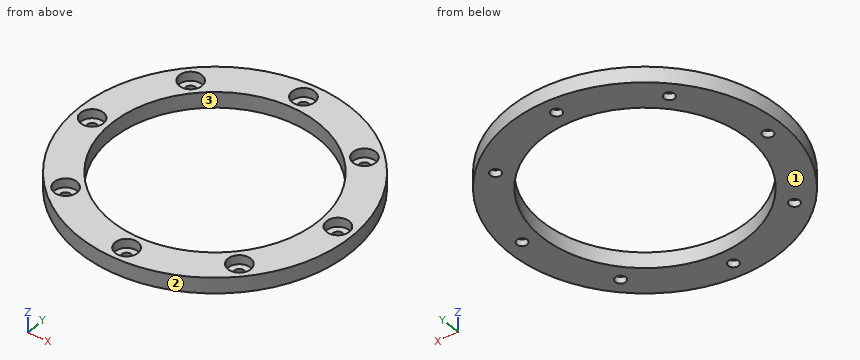
Autodesk Inventor part; units mm, degrees
ref_plane "YZ Plane" through (0, 0, 0) normal (1, 0, 0) x (0, 1, 0)
ref_plane "XZ Plane" through (0, 0, 0) normal (0, 1, 0) x (-1, 0, 0)
ref_plane "XY Plane" through (0, 0, 0) normal (0, 0, 1) x (1, 0, 0)
sketch "Sketch1" plane through (0, 0, 0) normal (0, 0, 1) x (1, 0, 0)
  circle A0 centre (0, 0) radius 125
  circle A1 centre (0, 0) radius 164.5
  dimension "d0" = 39.5
  dimension "d1" = 250
extrude "Extrusion1" add sketch "Sketch1" along normal blind 41
sketch "Sketch2" plane through (0, 0, 41) normal (0, 0, 1) x (1, 0, 0)
  circle A0 centre (0, 0) radius 164.5 construction
  circle A1 centre (0, 0) radius 125 construction
  line L0 (0, 164.5) -> (0, 125) construction
  circle A2 centre (0, 144.75) radius 6.25
  dimension "d4" = 12.5
extrude "Extrusion2" cut sketch "Sketch2" against normal through all
sketch "Sketch3" plane through (0, 0, 41) normal (0, 0, 1) x (1, 0, 0)
  circle A0 centre (0, 144.75) radius 6.25
  circle A1 centre (0, 144.75) radius 13.75
  point P0 (0, 0)
  dimension "d10" = 27.5
extrude "Extrusion3" cut sketch "Sketch3" against normal blind 11
pattern_circular "Circular Pattern1" count 8 over 360 about axis through (0, 0, 0) along (0, 0, 1) of "Extrusion2", "Extrusion3"
sketch "Sketch4" plane through (0, 0, 0) normal (0, 0, -1) x (-1, 0, 0)
  circle A0 centre (0, 0) radius 164.5
  circle A1 centre (0, 0) radius 169.5
  dimension "d13" = 5
extrude "Extrusion4" add sketch "Sketch4" against normal blind 10
sketch "Sketch5" plane through (0, 0, 0) normal (1, 0, 0) x (0, 1, 0)
  line L0 (164.5, 10) -> (-164.5, 10)
  line L1 (164.5, 41) -> (-164.5, 41)
  line L2 (169.5, 10) -> (-169.5, 10)
  line L3 (-169.5, 0) -> (169.5, 0)
  line L4 (164.5, 41) -> (164.5, 10)
  line L5 (164.5, 10) -> (164.5, 41)
  line L6 (169.5, 10) -> (169.5, 0)
  line L7 (169.5, 0) -> (169.5, 10)
  line L8 (-169.5, 0) -> (169.5, 0)
  line L9 (-169.5, 0) -> (-169.5, 10)
  line L10 (-169.5, 0) -> (-169.5, 10)
  line L11 (-164.5, 10) -> (-164.5, 41)
  line L12 (164.5, 22) -> (-164.5, 22)
  line L13 (-164.5, 10) -> (-164.5, 41)
  point P0 (0, 0)
  dimension "d17" = 22
extrude "Extrusion5" cut sketch "Sketch5" along normal through all both and the other way through all contours L2 L6 L3 L9 L0 | L0 L11 L12 L4
equation "\"d1\" = Вал_ось_диаметр_НОС"
equation "\"BendRadius\" = Thickness"
equation "\"BendReliefWidth\" = Thickness"
equation "\"BendReliefDepth\" = 0.5 * Thickness"
equation "\"CornerReliefSize\" = 4 * Thickness"
equation "\"MinimumRemnant\" = 2 * Thickness"
equation "\"TransitionRadius\" = BendRadius"
equation "\"JacobiRadiusSize\" = BendRadius"
equation "\"GapSize\" = Thickness"
properties part number "ДМФ 01 31.2 Барабан Опорное кольцо НОС"
The model under review builds one solid part; all positions refer to its coordinate system, in mm. Face numbers are marked on the shaded views. Round coordinates to 2 decimals unless told otherwise and drop trailing zeros. Order: outer loops, then holes, each group sorted by start corner. A loop starts at its lowest first (then second) coordinate and runs counter-clockwise, first axis right, second up. Notation, with made-up numbers: (13.5, 68) -> (26.5, 68) arc R20 ccw to (26.5, 74) -> close; hole circle Ø9 at (-13.75, 9.5). An arc over 180 degrees is marked (long way). Return JSON: item names as keys, results as strings.
1. Take a section at A-A (x = 0). Write out the cut boundary in (y, z).
Answer block:
{"outline": "(-164.5, 22) -> (-151, 22) -> (-151, 30) -> (-158.5, 30) -> (-158.5, 41) -> (-164.5, 41) -> close; (-138.5, 22) -> (-125, 22) -> (-125, 41) -> (-131, 41) -> (-131, 30) -> (-138.5, 30) -> close; (125, 22) -> (138.5, 22) -> (138.5, 30) -> (131, 30) -> (131, 41) -> (125, 41) -> close; (151, 22) -> (164.5, 22) -> (164.5, 41) -> (158.5, 41) -> (158.5, 30) -> (151, 30) -> close"}
2. Insertion check: P1, Ø20, axis at x = -102.35, y = -102.35, coming from the +Z side; P2, Ø3, axis at x = -129, z = 28, coming from the -Y side; P3, Ø3, axis at y = 125, z = 28, coming from the +X side. Each pin has a flat end and moves straight along its axis. Give the tip position at first contact, or say it passes through.
Answer block:
{"P1": "stops at z = 30", "P2": "stops at y = -103.94", "P3": "stops at x = 108.66"}
3. Take a section at C-C (x = -49). Write out the cut boundary in (y, z), then the cut area to 3 significant figures.
Answer block:
{"outline": "(-157.03, 22) -> (-115, 22) -> (-115, 41) -> (-157.03, 41) -> close; (115, 22) -> (157.03, 22) -> (157.03, 41) -> (115, 41) -> close", "area": "1,600 mm²"}
4. Take a section at D-D (y = -144.75). Write out the cut boundary in (x, z), then the cut area to 3 significant figures.
Answer block:
{"outline": "(-78.15, 22) -> (-6.25, 22) -> (-6.25, 30) -> (-13.75, 30) -> (-13.75, 41) -> (-78.15, 41) -> close; (6.25, 22) -> (78.15, 22) -> (78.15, 41) -> (13.75, 41) -> (13.75, 30) -> (6.25, 30) -> close", "area": "2,570 mm²"}
5. For L1, parallel to Y at x = 0, z = 26.75; L2, parallel to Y at x = 95.5, z = 37.5; L3, parallel to X at y = 103.5, z = 24.25, list the stretches that pass through material, from the lowest coordinate up. Write a range as [from, to].
Answer block:
{"L1": "y = [-164.5, -151], [-138.5, -125], [125, 138.5], [151, 164.5]", "L2": "y = [-133.94, -114.27], [-90.43, -80.65], [80.65, 90.43], [114.27, 133.94]", "L3": "x = [-127.86, -108.5], [-96.21, -70.09], [70.09, 96.21], [108.5, 127.86]"}
6. The part is to be moulded in two halves that separate along Y. For the marked faces 1, 2 and 3, say which applies: +Y half, -Y half, draft (parallel to the pull), parting line (faces both ways), or undercut.
Answer block:
{"face 1": "draft", "face 2": "parting line", "face 3": "undercut"}
